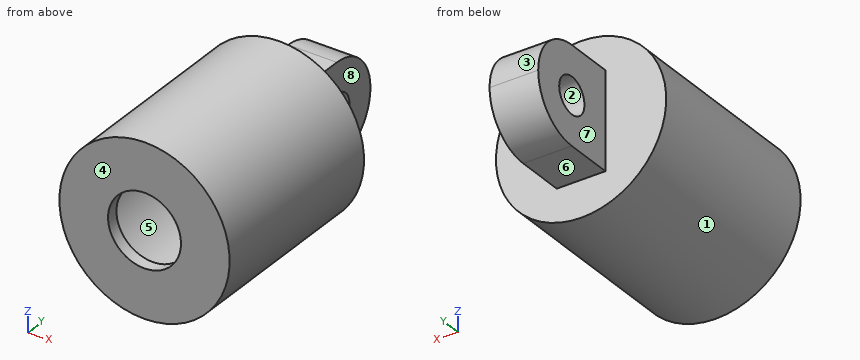
Autodesk Inventor part; units mm, degrees
ref_plane "YZ Plane" through (0, 0, 0) normal (1, 0, 0) x (0, 1, 0)
ref_plane "XZ Plane" through (0, 0, 0) normal (0, 1, 0) x (-1, 0, 0)
ref_plane "XY Plane" through (0, 0, 0) normal (0, 0, 1) x (1, 0, 0)
sketch "Sketch1" plane through (0, 0, 0) normal (1, 0, 0) x (0, 1, 0)
  line L0 (-50.8, 44.45) -> (50.8, 44.45)
  line L1 (50.8, 44.45) -> (50.8, 41.275)
  line L2 (-50.8, 41.275) -> (-50.8, 44.45)
  line L3 (-50.8, 44.45) -> (-47.1714, 41.275) construction
  line L4 (50.8, 41.275) -> (-50.8, 41.275)
  line L5 (50.8, 44.45) -> (47.1714, 41.275) construction
  line L6 (-71.12, 0) -> (71.12, 0)
  point P0 (0, 0)
revolve "Revolution1" add sketch "Sketch1" angle 360 about axis through (0, -10, 0) along (0, 1, 0)
sketch "Sketch2" plane through (0, 50.8, 0) normal (0, 1, 0) x (1, 0, 0)
  circle A0 centre (0, 0) radius 44.45
extrude "Extrusion1" add sketch "Sketch2" against normal blind 6.35
sketch "Sketch3" plane through (0, -50.8, 0) normal (0, -1, 0) x (1, 0, 0)
  circle A0 centre (0, 0) radius 44.45
extrude "Extrusion2" add sketch "Sketch3" against normal blind 6.35
sketch "Sketch4" plane through (0, -50.8, 0) normal (0, -1, 0) x (1, 0, 0)
  circle A0 centre (0, 0) radius 44.45
  circle A1 centre (0, 0) radius 19.05
extrude "Extrusion3" cut sketch "Sketch4" against normal blind 12.7 contours A1
sketch "Sketch5" plane through (0, 50.8, 0) normal (0, 1, 0) x (1, 0, 0)
  line L0 (-25.4, 25.4) -> (25.4, 25.4)
  line L1 (25.4, 25.4) -> (25.4, -25.4)
  line L2 (25.4, -25.4) -> (-25.4, -25.4)
  line L3 (-25.4, -25.4) -> (-25.4, 25.4)
  line L4 (-25.4, 25.4) -> (25.4, -25.4) construction
  line L5 (25.4, 25.4) -> (-25.4, -25.4) construction
  line L6 (-12.7, 25.4) -> (12.7, 25.4)
  line L7 (12.7, 25.4) -> (12.7, -25.4)
  line L8 (12.7, -25.4) -> (-12.7, -25.4)
  line L9 (-12.7, -25.4) -> (-12.7, 25.4)
  line L10 (-12.7, 25.4) -> (12.7, -25.4) construction
  line L11 (12.7, 25.4) -> (-12.7, -25.4) construction
  point P0 (0, 0)
  dimension "d9" = 50.8
  dimension "d10" = 50.8
extrude "Extrusion6" add sketch "Sketch5" along normal blind 50.8 contours L0 L7 L2 L9
fillet "Fillet2" radius 25.4 2 edges at (0, 101.6, 25.4) (0, 101.6, -25.4)
sketch "Sketch7" plane through (12.7, 50.8, 25.4) normal (1, 0, 0) x (0, 0, -1)
  arc A0 (50.8, 25.4) -> (0, 25.4) centre (25.4, 25.4) ccw
  circle A1 centre (25.4, 25.4) radius 9.525
  point P0 (25.4, -50.8)
  dimension "d20" = 19.05
extrude "Extrusion7" cut sketch "Sketch7" against normal blind 50.8
properties part number "shock absorber top"
Could you check a few things on this model? Use its own coordinates, in mm. Face numbers are marked on the shaded views. A direction names the side the tool comes from. Round coordinates to 2 decimals unless told otherwise and drop trailing zeros. Write each loop counter-clockwise with the first axis right and the second up, starting at its lowest first coordinate (ties: lowest second). Pieces come first, ordered by that corner, then holes.
(1) Which directions (+Z, -Z, +X, -X, +Y, -Y) give clear straight access to the entire face, cutting with the end or side of a thin tool? Please do the marked faces 5, 6, 7 and 8.
Findings below:
face 5: none
face 6: -Z, +X, -X, +Y
face 7: +Z, -Z, -X, +Y
face 8: +Z, -Z, +X, +Y
(2) Suppose I cut it at C-C on y = 81. Write out the boundary of the cut face in (x, z), and give its area (3 significant figures).
Findings below:
outline: (-12.7, -24.94) - (12.7, -24.94) - (12.7, -8.23) - (-12.7, -8.23) - close; (-12.7, 8.23) - (12.7, 8.23) - (12.7, 24.94) - (-12.7, 24.94) - close
area: 849 mm2
(3) Suppose I cut it at D-D on z = 37. Write out the boundary of the cut face in (x, y), and give its area (3 significant figures).
Findings below:
outline: (-24.63, -50.8) - (24.63, -50.8) - (24.63, 50.8) - (-24.63, 50.8) - close; hole (-18.29, -44.45) - (18.29, -44.45) - (18.29, 44.45) - (-18.29, 44.45) - close
area: 1,750 mm2
(4) Suppose I cut it at A-A on z = 3. Write out the boundary of the cut face in (x, y), and give its area (3 significant figures).
Findings below:
outline: (-44.35, -50.8) - (-18.81, -50.8) - (-18.81, -44.45) - (-41.17, -44.45) - (-41.17, 44.45) - (41.17, 44.45) - (41.17, -44.45) - (18.81, -44.45) - (18.81, -50.8) - (44.35, -50.8) - (44.35, 50.8) - (12.7, 50.8) - (12.7, 67.16) - (-12.7, 67.16) - (-12.7, 50.8) - (-44.35, 50.8) - close; (-12.7, 85.24) - (12.7, 85.24) - (12.7, 101.42) - (-12.7, 101.42) - close
area: 2,280 mm2
(5) If I drill on probe 1 along Z at (x, y) = (-4, 76); probe 2 along Z at (x, y) = (0, -47); probe 3 along X at (y, z) = (27.5, 0) (3 decimals), over which ranges is the centre line in solid material (lowest first)?
Findings below:
probe 1: z = -25.4 to -9.52, 9.52 to 25.4
probe 2: z = -44.45 to -19.05, 19.05 to 44.45
probe 3: x = -44.45 to -41.275, 41.275 to 44.45
(6) Thinking about a two-plate mould opening in Y: for the marked faces 1, 2, 3 and 4, which applies, +Y half, -Y half, draft (parallel to the pull), parting line (faces both ways), or undercut?
Findings below:
face 1: draft
face 2: undercut
face 3: +Y half
face 4: -Y half
(7) For pin 1 (6 mm diameter, centred on y = 83.5, z = -23, fed in from -X); pin 2 (2 mm diameter, centred on x = 4.5, z = 13.5, fed in from +Y); pin 3 (3 mm diameter, centred on x = 2, z = 13, fed in from +Y), each with a flat end and sliding along its axis, tell me the tip position at first contact or that it passes through.
Findings below:
pin 1: stops at x = -12.7
pin 2: stops at y = 98.31
pin 3: stops at y = 98.85
